For this review, use the dimensioned drawing (mm, ordinates from the lowest corner) and the shaded views. Coordinates: 2 decimals unless noted, no trailing zeros. Loops run counter-clockwise (first coordinate to the right, second up) from the corner with the lowest first, then second, coordinate; pieces in that order, holes last.
1. Clearance check with flat-ended pins moving along their axes: P1, Ø3, axis at x = 30, y = 11.5, coming from the -Z side; P2, Ø0.9, axis at x = 25.5, z = 1, coming from the -Y side; P3, Ø0.6, axis at y = 1, z = 2, coming from the -X side. State where each tip first meets the part, or that it passes through.
2. Take a section at B-B, the plane x = 26.5. State the section outline as (y, z) points.
3. Take a section at A-A, the plane z = 1.45. State the section outline as (x, y) points, then the cut area to 3 significant figures.
4. To check wall thickness, follow probe 1 along X at (y, z) = (1.5, 1.4); probe 2 along Y at (x, z) = (48, 1.4); probe 3 along X at (y, z) = (17.75, 2.7). State the ranges of each line that lie inside material, in increasing order.
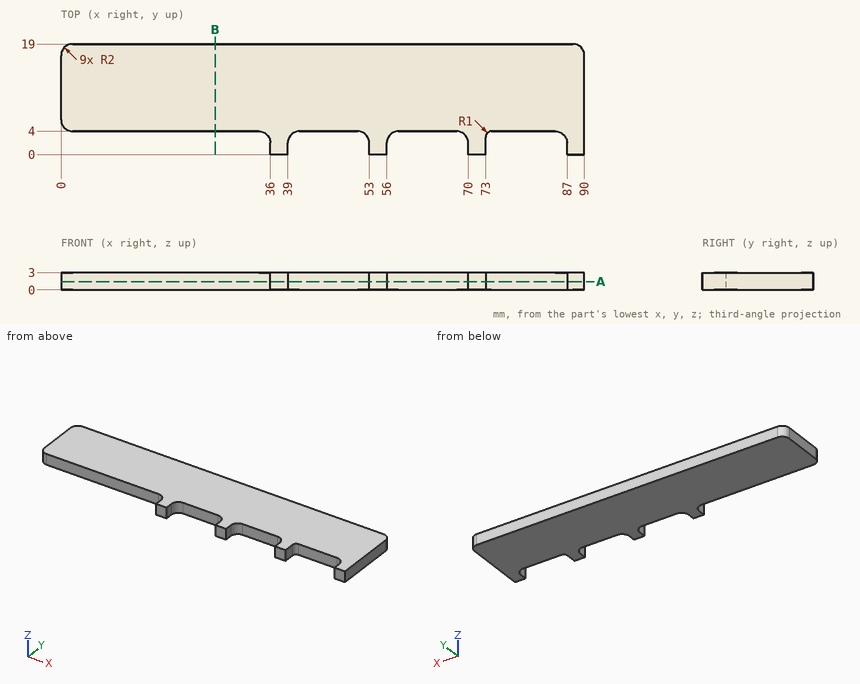
Results list:
1. P1: stops at z = 0
1. P2: stops at y = 4
1. P3: stops at x = 36
2. outline: (4, 0) - (19, 0) - (19, 3) - (4, 3) - close
3. outline: (0, 6) arc R2 ccw to (2, 4) - (34, 4) arc R2 cw to (36, 2) - (36, 0) - (39, 0) - (39, 2) arc R2 cw to (41, 4) - (51, 4) arc R2 cw to (53, 2) - (53, 0) - (56, 0) - (56, 2) arc R2 cw to (58, 4) - (68, 4) arc R2 cw to (70, 2) - (70, 0) - (73, 0) - (73, 3) arc R1 cw to (74, 4) - (85, 4) arc R2 cw to (87, 2) - (87, 0) - (90, 0) - (90, 17) arc R2 ccw to (88, 19) - (2, 19) arc R2 ccw to (0, 17) - close
3. area: 1,400 mm2
4. probe 1: x = 36 to 39, 53 to 56, 70 to 73, 87 to 90
4. probe 2: y = 4 to 19
4. probe 3: x = 0.15 to 89.85
